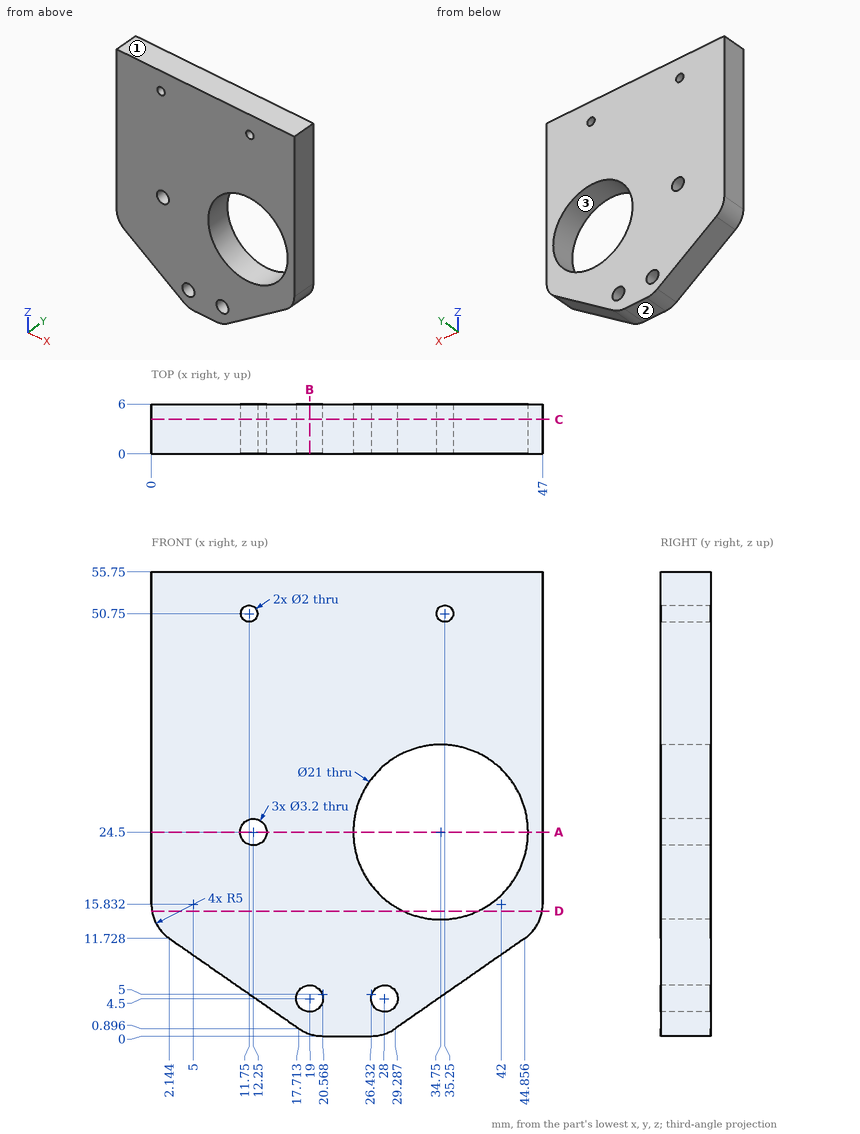
Check sheet for the drawn part. Datum: minimum x, y, z corner. Units: mm. Round coordinates to 2 decimals unless told otherwise and drop trailing zeros. Loops run counter-clockwise (first coordinate to the right, second up) from the corner with the lowest first, then second, coordinate; pieces in that order, holes last. Notation, with made-up numbers: (67.5, 16.25) - (115.5, 16.25) arc R24 cw to (115.5, 47.25) - close; hole circle Ø6 at (29, 5). An arc over 180 degrees is marked (long way). Answer as a JSON object with one key per item and string values. Group by question number.
Q1. Mould release check, pull along Z, two halves, no side actions. Record for the marked faces 1, 2 and 3: released by +Z, released by -Z, zero draft, split by the parting line, or undercut.
Q2. Sectioned sample at D-D, the plane z = 15. Enter the section's corners in (x, y).
Q3. Scan lines: line 1 along Z through (x, y) = (12, 3.3); line 2 along Z through (x, y) = (28, 3.75); line 3 along X through (y, z) = (1.8, 4.5) (1 decimal). Record each from-to range of solid material in increasing order. Write a range as [from, to].
Q4. Sectioned sample at B-B, the plane x = 19. Enter the section's corners in (y, z), plus the area to 3 significant figures.
Q5. Sectioned sample at A-A, the plane z = 24.5. Enter the section's corners in (x, y), plus the area to 3 significant figures.
Q6. Sectioned sample at C-C, the plane y = 4.15. Count the separate pieces of the cut face and the enclosed holes in it, plus the area to 3 significant figures.
Solution:
{
 "1": {"face 1": "released by +Z", "face 2": "released by -Z", "face 3": "undercut"},
 "2": {"outline": "(0.07, 0) - (30.28, 0) - (30.28, 6) - (0.07, 6) - close; (39.22, 0) - (46.93, 0) - (46.93, 6) - (39.22, 6) - close"},
 "3": {"line 1": "z = [4.87, 22.92], [26.08, 49.78], [51.72, 55.75]", "line 2": "z = [0.25, 2.9], [6.1, 16.46], [32.54, 55.75]", "line 3": "x = [12.5, 17.4], [20.6, 26.4], [29.6, 34.5]"},
 "4": {"outline": "(0, 0.25) - (6, 0.25) - (6, 2.9) - (0, 2.9) - close; (0, 6.1) - (6, 6.1) - (6, 55.75) - (0, 55.75) - close", "area": "314 mm²"},
 "5": {"outline": "(0, 0) - (10.65, 0) - (10.65, 6) - (0, 6) - close; (13.85, 0) - (24.25, 0) - (24.25, 6) - (13.85, 6) - close; (45.25, 0) - (47, 0) - (47, 6) - (45.25, 6) - close", "area": "137 mm²"},
 "6": {"separate pieces": "1", "enclosed holes": "6", "area": "1,990 mm²"}
}
